Model file for the job. Use its own axes, mm. Face numbers are marked on the shaded views. A direction names the side the tool comes from. Round coordinates to 2 decimals unless told otherwise and drop trailing zeros. Order: outer loops, then holes, each group sorted by start corner. A loop starts at its lowest first (then second) coordinate and runs counter-clockwise, first axis right, second up. Notation, with made-up numbers: (75.5, 27) -> (90.5, 27) arc R30 cw to (90.5, 64) -> close; hole circle Ø11 at (77.25, 43). An arc over 180 degrees is marked (long way). Use CSV: the item, a comma, the result in double quotes.
```python
from build123d import *

# Parameters (mm, degrees)
BOSS_EXTRUDE1_DEPTH = 3
SKETCH2_R           = 2.75
CUT_EXTRUDE3_DEPTH  = 163.815846895
BOSS_EXTRUDE3_DEPTH = 12.7
BOSS_EXTRUDE4_START = 8
SKETCH8_R           = 2.75
BOSS_EXTRUDE4_DEPTH = 8
SKETCH9_W           = 4
SKETCH9_H           = 15.601931027
BOSS_EXTRUDE5_DEPTH = 12.7
SKETCH10_R          = 2.75
CUT_EXTRUDE4_DEPTH  = 110.875
FILLET3_R           = 5
SKETCH11_R          = 5
CUT_EXTRUDE5_DEPTH  = 15.875
FILLET4_R           = 2
FILLET5_R           = 3
FILLET7_R           = 2


with BuildPart() as part:
    # Sketch1 → Boss-Extrude1 (new body)
    with BuildSketch(Plane(origin=(0, 0, 0), x_dir=(1, 0, 0), z_dir=(0, 1, 0))):
        Polygon((0, 0), (120, 0), (120, -47), (4, -96.23907868), (4, -110), (0, -110), align=None)
    extrude(amount=BOSS_EXTRUDE1_DEPTH)

    # Sketch2 → Cut-Extrude3 (cut, through all)
    with BuildSketch(Plane(origin=(0, 3, 0), x_dir=(1, 0, 0), z_dir=(0, 1, 0))):
        with Locations(Location((112, -7.5, 0), (0, 0, 270))):
            Circle(SKETCH2_R)
        with Locations(Location((112, -42.5, 0), (0, 0, 270))):
            Circle(SKETCH2_R)
        Polygon((104, -8), (104, -45.10071404), (8, -85.850296396), (8, -8), align=None)
    extrude(amount=-CUT_EXTRUDE3_DEPTH, mode=Mode.SUBTRACT)

    # Sketch7 → Boss-Extrude3 (add)
    with BuildSketch(Plane(origin=(0, 3, 0), x_dir=(1, 0, 0), z_dir=(0, 1, 0))):
        Polygon((118, -45.676228878), (3.218537743, -94.398068973), (4, -96.23907868), (120, -47), (120, 0), (3.218537743, 0), (3.218537743, -2), (118, -2), align=None)
    extrude(amount=BOSS_EXTRUDE3_DEPTH)

    # Sketch8 → Boss-Extrude4 (add)
    # profile 1 of 2: a face of its own
    with BuildSketch(Plane(origin=(0, 3, 0), x_dir=(1, 0, 0), z_dir=(0, 1, 0)).offset(BOSS_EXTRUDE4_START)):
        with BuildLine():
            Line((112, -12.5), (118, -12.5))
            Line((118, -12.5), (118, -2))
            Line((118, -2), (107, -2))
            Line((107, -2), (107, -7.5))
            ThreePointArc((107, -7.5), (108.464466094, -11.035533906), (112, -12.5))
        make_face()
        with Locations(Location((112, -7.5, 0), (0, 0, 270))):
            Circle(SKETCH8_R, mode=Mode.SUBTRACT)
    # profile 2 of 2: a face of its own
    with BuildSketch(Plane(origin=(0, 3, 0), x_dir=(1, 0, 0), z_dir=(0, 1, 0)).offset(BOSS_EXTRUDE4_START)):
        with BuildLine():
            Line((112, -37.5), (118, -37.5))
            Line((118, -37.5), (118, -45.676228878))
            Line((118, -45.676228878), (107, -50.345451856))
            Line((107, -50.345451856), (107, -42.5))
            ThreePointArc((107, -42.5), (108.464466094, -38.964466094), (112, -37.5))
        make_face()
        with Locations(Location((112, -42.5, 0), (0, 0, 270))):
            Circle(SKETCH8_R, mode=Mode.SUBTRACT)
    extrude(amount=-BOSS_EXTRUDE4_DEPTH)

    # Sketch9 → Boss-Extrude5 (add)
    with BuildSketch(Plane(origin=(0, 3, 0), x_dir=(1, 0, 0), z_dir=(0, 1, 0))):
        with Locations((2, -7.800965514)):
            Rectangle(SKETCH9_W, SKETCH9_H)
        with Locations((2, -102.199034487)):
            Rectangle(SKETCH9_W, SKETCH9_H)
    extrude(amount=BOSS_EXTRUDE5_DEPTH)

    # Sketch10 → Cut-Extrude4 (cut)
    with BuildSketch(Plane(origin=(4, 0, 0), x_dir=(0, 0, -1), z_dir=(1, 0, 0))):
        with Locations((-8.800965513, 9.35)):
            Circle(SKETCH10_R)
        with Locations((-103.11953934, 9.35)):
            Circle(SKETCH10_R)
    extrude(amount=-CUT_EXTRUDE4_DEPTH, mode=Mode.SUBTRACT)

    # Fillet3
    fillet3_edges = [part.edges().sort_by_distance(p)[0] for p in [
        (120, 7.85, 0),
        (120, 7.85, 47),
        (2, 3, 15.601931027),
        (2, 15.7, 15.601931027),
        (2, 15.7, 110),
        (8, 1.5, 8),
        (104, 1.5, 8),
        (104, 1.5, 45.10071404),
        (8, 1.5, 85.850296396),
        (118, 13.35, 2),
        (118, 13.35, 45.676228878),
    ]]
    fillet(fillet3_edges, radius=FILLET3_R)

    # Sketch11 → Cut-Extrude5 (cut)
    with BuildSketch(Plane(origin=(0, 3, 0), x_dir=(1, 0, 0), z_dir=(0, 1, 0))):
        with Locations(Location((112, -25, 0), (0, 0, 270))):
            Circle(SKETCH11_R)
    extrude(amount=-CUT_EXTRUDE5_DEPTH, mode=Mode.SUBTRACT)

    # Fillet4
    fillet4_edges = [part.edges().sort_by_distance(p)[0] for p in [
        (4, 7.85, 96.23907868),
        (4, 9.35, 2),
    ]]
    fillet(fillet4_edges, radius=FILLET4_R)

    # Fillet5
    fillet5_edges = [part.edges().sort_by_distance(p)[0] for p in [
        (107, 7, 50.345451856),
        (118, 7, 37.5),
        (118, 7, 12.5),
        (107, 7, 2),
    ]]
    fillet(fillet5_edges, radius=FILLET5_R)

    # Fillet7
    fillet7_edges = [part.edges().sort_by_distance(p)[0] for p in [
        (0, 7.85, 0),
        (3.218537743, 9.35, 94.398068973),
    ]]
    fillet(fillet7_edges, radius=FILLET7_R)


solid = part.part
```
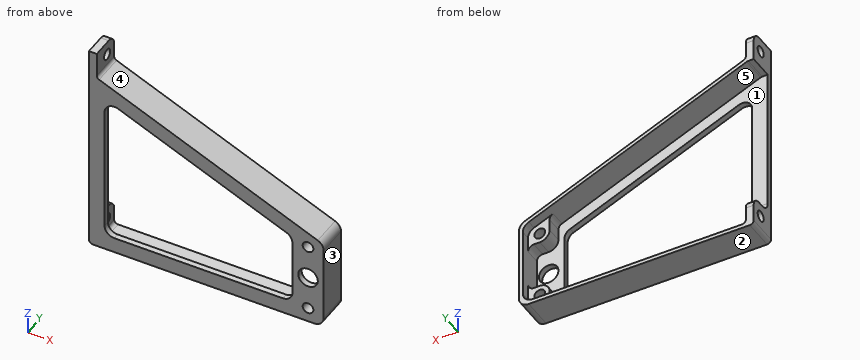
Q1. Cut at B-B (x = 18). Give the cut face in (y, z), plus the area to 3 significant figures.
From the geometry:
outline,"(0, 0) -> (15.7, 0) -> (15.7, 2) -> (3, 2) -> (3, 8) -> (0, 8) -> close; (0, 81.61) -> (3, 81.61) -> (3, 88.12) -> (15.7, 88.12) -> (15.7, 90.3) -> (0, 90.3) -> close"
area,"103 mm²"
Q2. Probe line 1 along X through (y, z) = (1.25, 25); line 2 along X through (y, z) = (6.75, 7.5); line 3 along Z through (x, y) = (114.5, 1). List the from-to ranges inside material, lowest first.
From the geometry:
line 1,"x = 0 to 8, 104 to 107, 117 to 120"
line 2,"x = 0 to 4, 107 to 109.25, 114.75 to 120"
line 3,"z = 0 to 6.35, 8.65 to 20.67, 29.33 to 41.35, 43.65 to 49.33"
Q3. Cut at C-C (y = 9.35). State how many separate pieces and enclosed holes the cut face has, plus the area to 3 significant figures.
From the geometry:
separate pieces,"3"
enclosed holes,"2"
area,"824 mm²"
Q4. Pin check, flat tips, straight feed: pin 1 (4.5 mm diameter, centred on x = 112, z = 7.5, fed in from +Y); pin 2 (1 mm diameter, centred on x = 77, y = 8.5, fed in from +Z); pin 3 (6.5 mm diameter, centred on x = 78, y = 7.5, fed in from +Z); pin 4 (6 mm diameter, centred on y = 8, z = 102.5, fed in from +X). Stop position of each tip, or through.
From the geometry:
pin 1,"passes through"
pin 2,"stops at z = 65.46"
pin 3,"stops at z = 66.21"
pin 4,"stops at x = 4"
Q5. Which spindle directions (+Z, -Z, +X, -X, +Y, -Y) get a long thin tool onto all of the face, cutting with end or side? Do the marked faces 1 and 2. Say none if no direction does.
From the geometry:
face 1,"+Y"
face 2,"-Z, +X, -X, +Y, -Y"
Q6. Cut at A-A (z = 25). Give the cut face in (x, y), plus the area to 3 significant figures.
From the geometry:
outline,"(0, 0) -> (8, 0) -> (8, 3) -> (0, 3) -> close; (104, 0) -> (107, 0) -> (107, 3) -> (104, 3) -> close; (117, 0) -> (120, 0) -> (120, 15.7) -> (118, 15.7) -> (118, 3) -> (117, 3) -> close"
area,"67.4 mm²"
Q7. Mould opens along Z. For the marked faces 3, 4 and 5 say: +Z half, -Z half, draft (parallel to the pull), parting line (faces both ways), or undercut.
From the geometry:
face 3,"draft"
face 4,"+Z half"
face 5,"undercut"
Q8. Cut at D-D (z = 63). Give the cut face in (x, y), plus the area to 3 significant figures.
From the geometry:
outline,"(0, 0) -> (8, 0) -> (8, 3) -> (0, 3) -> close; (61.83, 0) -> (82.31, 0) -> (82.31, 15.7) -> (77.19, 15.7) -> (77.19, 3) -> (61.83, 3) -> close"
area,"150 mm²"
